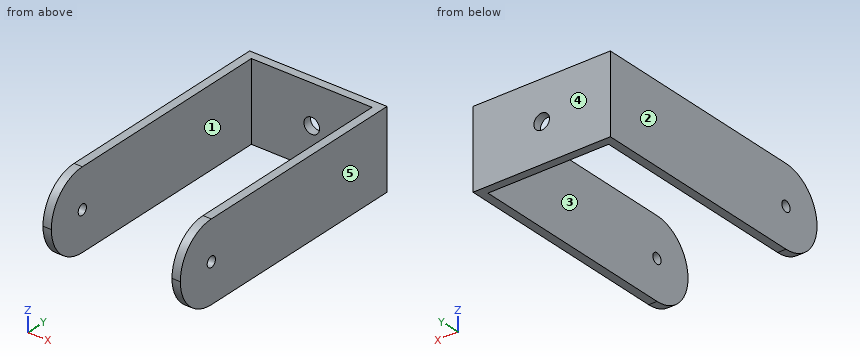
from build123d import *

# Parameters (mm, degrees)
BOSS_EXTRUDE1_DEPTH = 75
SKETCH2_R           = 7.5
CUT_EXTRUDE1_DEPTH  = 8
SKETCH3_R           = 5
CUT_EXTRUDE2_DEPTH  = 134
FILLET1_R           = 37.5


with BuildPart() as part:
    # Sketch1 → Boss-Extrude1 (new body)
    with BuildSketch(Plane.XY):
        Polygon((124, -250), (132, -250), (132, 0), (0, 0), (0, -250), (8, -250), (8, -8), (124, -8), align=None)
    extrude(amount=BOSS_EXTRUDE1_DEPTH)

    # Sketch2 → Cut-Extrude1 (cut)
    with BuildSketch(Plane(origin=(0, 0, 0), x_dir=(1, 0, 0), z_dir=(0, 1, 0))):
        with Locations(Location((66, -37.5, 0), (0, 0, 270))):
            Circle(SKETCH2_R)
    extrude(amount=-CUT_EXTRUDE1_DEPTH, mode=Mode.SUBTRACT)

    # Sketch3 → Cut-Extrude2 (cut)
    with BuildSketch(Plane(origin=(132, 0, 0), x_dir=(0, 0, -1), z_dir=(1, 0, 0))):
        with Locations(Location((-37.5, -212.5, 0), (0, 0, 90))):
            Circle(SKETCH3_R)
    extrude(amount=-CUT_EXTRUDE2_DEPTH, mode=Mode.SUBTRACT)

    # Fillet1
    fillet1_edges = [part.edges().sort_by_distance(p)[0] for p in [
        (128, -250, 75),
        (4, -250, 75),
        (4, -250, 0),
        (128, -250, 0),
    ]]
    fillet(fillet1_edges, radius=FILLET1_R - 0.0001)  # a hair under: the kernel refuses the full size


solid = part.part
Can you work these out from the model? Positions are in its coordinate system, mm. Face numbers are marked on the shaded views. A direction names the side the tool comes from. Coordinates: 2 decimals unless noted, no trailing zeros. Write each loop counter-clockwise with the first axis right and the second up, starting at its lowest first coordinate (ties: lowest second). Pieces come first, ordered by that corner, then holes. Notation, with made-up numbers: (35, 70) - (74, 70) arc R15 ccw to (74, 87) - close; hole circle Ø7 at (35.25, -17). An arc over 180 degrees is marked (long way). Return JSON: item names as keys, results as strings. Group by question number.
Item 1: If we section it at A-A (x = 66): Write out the boundary of the cut face in (y, z).
Item 2: If we section it at D-D (x = 120.5): Write out the boundary of the cut face in (y, z), then the cut area to 3 significant figures.
Item 3: Please list where these lines run through material, in increasing order: probe 1 along X at (y, z) = (-195.5, 13.5); probe 2 along Z at (x, y) = (129.25, -212.5); probe 3 along Y at (x, z) = (125, 37).
Item 4: Which directions (+Z, -Z, +X, -X, +Y, -Y) give clear straight access to the entire face, cutting with the end or side of a thin tool? Please do the marked faces 1 and 2.
Item 5: We'd pull the mould along X, two halves only. Please class the marked faces 3, 4 and 5: pulls with the +X half, pulls with the -X half, needs draft (parallel to the pull), parting line crosses it, or undercut.
Item 6: If we section it at B-B (y = -104): Write out the boundary of the cut face in (x, z), then the cut area to 3 significant figures.
Item 7: I'm going to push a flat-ended pin straight in: pin 1 Ø12 at (x, z) = (88, 36) entering from -Y. Where does the tip first touch, or does it pass through?
Item 8: If we section it at C-C (z = 60): Write out the boundary of the cut face in (x, y), then the cut area to 3 significant figures.
Return value:
{
 "1": {"outline": "(-8, 0) - (0, 0) - (0, 30) - (-8, 30) - close; (-8, 45) - (0, 45) - (0, 75) - (-8, 75) - close"},
 "2": {"outline": "(-8, 0) - (0, 0) - (0, 75) - (-8, 75) - close", "area": "600 mm^2"},
 "3": {"probe 1": "x = 0 to 8, 124 to 132", "probe 2": "z = 0 to 32.5, 42.5 to 75", "probe 3": "y = -250 to -217.47, -207.53 to 0"},
 "4": {"face 1": "+Z, -Z, -Y", "face 2": "+Z, -Z, -X, +Y, -Y"},
 "5": {"face 3": "undercut", "face 4": "needs draft", "face 5": "pulls with the +X half"},
 "6": {"outline": "(0, 0) - (8, 0) - (8, 75) - (0, 75) - close; (124, 0) - (132, 0) - (132, 75) - (124, 75) - close", "area": "1,200 mm^2"},
 "7": {"pin 1": "stops at y = -8"},
 "8": {"outline": "(0, -242.5) - (8, -242.5) - (8, -8) - (124, -8) - (124, -242.5) - (132, -242.5) - (132, 0) - (0, 0) - close", "area": "4,810 mm^2"}
}
